```python
from build123d import *

# Parameters (mm, degrees)
SKETCH1_W           = 25.4
SKETCH1_H           = 12.7
SKETCH1_R           = 3
SKETCH1_R_2         = 3.175
BOSS_EXTRUDE1_DEPTH = 3.175
FILLET1_R           = 6.35


with BuildPart() as part:
    # Sketch1 → Boss-Extrude1 (new body)
    with BuildSketch(Plane(origin=(0, 0, 0), x_dir=(1, 0, 0), z_dir=(0, 1, 0))):
        with Locations((12.7, 6.35)):
            Rectangle(SKETCH1_W, SKETCH1_H)
        with Locations(Location((19.05, 6.35, 0), (0, 0, 270))):
            Circle(SKETCH1_R, mode=Mode.SUBTRACT)
        with Locations(Location((6.35, 6.35, 0), (0, 0, 270))):
            Circle(SKETCH1_R_2, mode=Mode.SUBTRACT)
    extrude(amount=BOSS_EXTRUDE1_DEPTH)

    # Fillet1
    fillet1_edges = [part.edges().sort_by_distance(p)[0] for p in [
        (25.4, 1.5875, 0),
        (25.4, 1.5875, -12.7),
        (0, 1.5875, -12.7),
        (0, 1.5875, 0),
    ]]
    fillet(fillet1_edges, radius=FILLET1_R - 0.0001)  # a hair under: the kernel refuses the full size


solid = part.part
```
The model under review builds one solid part; all positions refer to its coordinate system, in mm. Round coordinates to 2 decimals unless told otherwise and drop trailing zeros. Loops run counter-clockwise (first coordinate to the right, second up) from the corner with the lowest first, then second, coordinate; pieces in that order, holes last. Notation, with made-up numbers: (73.25, 12) -> (77.25, 12) arc R21 cw to (77.25, 44) -> close; hole circle Ø7 at (-39, -24). An arc over 180 degrees is marked (long way). Answer as a JSON object with one key per item and string values. Group by question number.
1) Mouldability with a two-part tool opening along Z and no side actions: class faces 1 (the face through (22.024, 1.565, -6.741)), 2 (the face through (1.81, 1.61, -1.91)), 3 (the face through (13, 0, -6)) as released by +Z, released by -Z, zero draft, split by the parting line, or undercut.
2) For line 1 (X direction, y = 1.9, z = -6.35) (3 decimals); line 2 (Z direction, x = 6.25, y = 2.15); line 3 (Z direction, x = 21, y = 1.1), list the stretches that pass through material, from the lowest coordinate up. Write a range as [from, to].
3) We need section A-A on y = 1.8. Give the number of separate pieces and of enclosed holes in the cut face, then the cut area to 3 significant figures.
4) We need section C-C on z = -8.5. Write out the cut boundary in (x, y) (3 decimals), then the cut area to 3 significant figures.
5) We need section B-B on z = -4.5. Write out the cut boundary in (x, y) (3 decimals).
Result set:
{
 "1": {"face 1": "undercut", "face 2": "released by +Z", "face 3": "zero draft"},
 "2": {"line 1": "[0, 3.175], [9.525, 16.05], [22.05, 25.4]", "line 2": "[-12.7, -9.52], [-3.18, 0]", "line 3": "[-12.39, -8.63], [-4.07, -0.31]"},
 "3": {"separate pieces": "1", "enclosed holes": "2", "area": "228 mm²"},
 "4": {"outline": "(0.375, 0) -> (4.014, 0) -> (4.014, 3.175) -> (0.375, 3.175) -> close; (8.686, 0) -> (16.958, 0) -> (16.958, 3.175) -> (8.686, 3.175) -> close; (21.142, 0) -> (25.025, 0) -> (25.025, 3.175) -> (21.142, 3.175) -> close", "area": "50.1 mm²"},
 "5": {"outline": "(0.275, 0) -> (3.77, 0) -> (3.77, 3.175) -> (0.275, 3.175) -> close; (8.93, 0) -> (16.688, 0) -> (16.688, 3.175) -> (8.93, 3.175) -> close; (21.412, 0) -> (25.125, 0) -> (25.125, 3.175) -> (21.412, 3.175) -> close"}
}
